from build123d import *

# Parameters (mm, degrees)
F0_R     = 9.525
F1_DEPTH = 76.2
F2_R     = 6.35
F3_T     = -3.175
F4_R     = 1.5875


with BuildPart() as f1:
    # F0 (on Top) → F1 (new body)
    with BuildSketch(Plane.XY):
        Circle(F0_R)
    extrude(amount=F1_DEPTH)

    # F2
    f2_edges = [f1.edges().sort_by_distance(p)[0] for p in [
        (-9.525, 0, 76.2),
    ]]
    fillet(f2_edges, radius=F2_R)

    # F3
    f3_openings = [f1.faces().sort_by_distance(p)[0] for p in [
        (0, 0, 0),
    ]]
    offset(amount=F3_T, openings=f3_openings)

    # F4
    f4_edges = [f1.edges().sort_by_distance(p)[0] for p in [
        (-6.35, 0, 0),
    ]]
    fillet(f4_edges, radius=F4_R)


solid = f1.part
Source: CAD feature listing. Evaluate the final solid. Frame: model axes, mm. A direction names the side the tool comes from. Give positions to 0.01 mm unless a question says otherwise; leave off trailing zeros. Write each loop counter-clockwise with the first axis right and the second up, starting at its lowest first coordinate (ties: lowest second). Pieces come first, ordered by that corner, then holes. Notation, with made-up numbers: (61, 78) -> (95, 78) arc R29 ccw to (95, 102) -> close; hole circle Ø11 at (72, -12.75). An arc over 180 degrees is marked (long way). Return JSON: item names as keys, results as strings. Group by question number.
1. Material intervals for line 1 (Y direction, x = 0, z = 22) (3 decimals); line 2 (X direction, y = -2.5, z = 39); line 3 (X direction, y = -0.75, z = 47), sorted ascending. Write a range as from..to.
2. Section A-A, the plane z = 25.5. Output: boundary loops of the cut face in (x, y) (3 decimals), then the cut area to 3 significant figures.
3. Pin query (flat end, axial travel): pin 1 Ø3 at (x, y) = (0.5, -1) entering from -Z (3 decimals); pin 2 Ø1 at (x, y) = (-4, -2.5) entering from +Z; pin 3 Ø4 at (y, z) = (-4.5, 44.5) entering from +X. Return the tip coordinate at first contact, or that it passes through.
4. Access query for faces 4 (the face through (0, 0, 76.2)), 5 (the face through (-0.8, 6.3, 35.2)). Directions: +Z, -Z, +X, -X, +Y, -Y. A direction counts if a zero-diameter tool reaches every point of the face in a straight line with its end or side. Return the directions, or none.
5. Mould query, pull axis Y, two halves, no side actions, for faces 1 (the face through (-2, 8, 0)), 2 (the face through (-7.559, -5.796, 34.436)), 3 (the face through (0, 0, 73.025)). Classes: +Y half, -Y half, draft (parallel to the pull), parting line (faces both ways), or undercut.
Determined:
{
 "1": {"line 1": "y = -9.525..-6.35, 6.35..9.525", "line 2": "x = -9.19..-5.84, 5.84..9.19", "line 3": "x = -9.5..-6.31, 6.31..9.5"},
 "2": {"outline": "circle Ø19.05 at (0, 0); hole circle Ø12.7 at (0, 0)", "area": "158 mm2"},
 "3": {"pin 1": "stops at z = 73.025", "pin 2": "stops at z = 76.11", "pin 3": "stops at x = 9.19"},
 "4": {"face 4": "+Z, +X, -X, +Y, -Y", "face 5": "-Z"},
 "5": {"face 1": "draft", "face 2": "parting line", "face 3": "undercut"}
}
